from build123d import *

# Parameters (mm, degrees)
SKETCH1_R           = 16.5
SKETCH1_R_2         = 15
BOSS_EXTRUDE1_DEPTH = 40
SKETCH3_W           = 4
SKETCH3_H           = 8
CUT_EXTRUDE1_DEPTH  = 47.308746474


with BuildPart() as part:
    # Sketch1 → Boss-Extrude1 (new, symmetric)
    with BuildSketch(Plane.XY):
        Circle(SKETCH1_R)
        Circle(SKETCH1_R_2, mode=Mode.SUBTRACT)
    extrude(amount=BOSS_EXTRUDE1_DEPTH, both=True)

    # Sketch3 → Cut-Extrude1 (cut, through all)
    with BuildSketch(Plane(origin=(0, 0, 0), x_dir=(0, 0, -1), z_dir=(1, 0, 0))):
        with Locations((-38, 0)):
            Rectangle(SKETCH3_W, SKETCH3_H)
    cut_extrude1 = extrude(amount=CUT_EXTRUDE1_DEPTH, mode=Mode.SUBTRACT)

    # Mirror1: Cut-Extrude1 across plane
    add(cut_extrude1.mirror(Plane.XY), mode=Mode.SUBTRACT)


solid = part.part
Here's how the part is built. I have some questions about the finished solid (model axes, mm). A direction names the side the tool comes from. Give positions to 0.01 mm unless a question says otherwise; leave off trailing zeros. Write each loop counter-clockwise with the first axis right and the second up, starting at its lowest first coordinate (ties: lowest second). Pieces come first, ordered by that corner, then holes. Notation, with made-up numbers: (-7, 18) -> (35, 18) arc R3 cw to (35, 22) -> close; hole circle Ø3 at (76, 57.25). An arc over 180 degrees is marked (long way). Use one line per item in the form item = value. Start each with the question number.
1. Imagine slicing it at B-B on y = 0. List the corners of the cut face in (x, z) for me, plus the area to 3 significant figures.
2. Imagine slicing it at C-C on z = -34. List the corners of the cut face in (x, y) for me, plus the area to 3 significant figures.
3. Imagine slicing it at A-A on x = 0. List the corners of the cut face in (y, z) for me, plus the area to 3 significant figures.
4. Thinking about a two-plate mould opening in X: for faces 1 (the face through (-14.985, 0.66, -0.56)), 2 (the face through (-15, -4, -40)), 3 (the face through (15.24, -6.32, 0.56)), which applies, +X half, -X half, draft (parallel to the pull), parting line (faces both ways), or undercut?
5. If I drill on L1, parallel to Y at x = 0, z = 2; L2, parallel to Y at x = -9, z = -4; L3, parallel to X at y = -2.5, z = 21.5, over which ranges is the centre line in solid material (lowest first)?
6. On a 3-axis mill with a long thin cutter (end or side, diameter ignored), from which of +Z, -Z, +X, -X, +Y, -Y can I reach the whole of each face in a straight line? I mean faces 4 (the face through (-15, -4, 40)), 5 (the face through (15, 4, 38)), 6 (the face through (15.5, -0.1, -36)). Say none if no direction works.
7. Will these pins go through, and if not, where does the flat tip stop? pin 1 Ø0.5 at (x, z) = (15.5, 37.5) entering from +Y; pin 2 Ø8 at (y, z) = (-8.5, 27.5) entering from +X; pin 3 Ø1.2 at (x, z) = (15.5, -37.5) entering from +Y.
Entries:
q1.outline = (-16.5, -40) -> (-15, -40) -> (-15, 40) -> (-16.5, 40) -> close; (15, -36) -> (16.5, -36) -> (16.5, 36) -> (15, 36) -> close
q1.area = 228 mm²
q2.outline = circle Ø33 at (0, 0); hole circle Ø30 at (0, 0)
q2.area = 148 mm²
q3.outline = (-16.5, -40) -> (-15, -40) -> (-15, 40) -> (-16.5, 40) -> close; (15, -40) -> (16.5, -40) -> (16.5, 40) -> (15, 40) -> close
q3.area = 240 mm²
q4.face_1 = undercut
q4.face_2 = draft
q4.face_3 = parting line
q5.L1 = -16.5 to -15, 15 to 16.5
q5.L2 = -13.83 to -12, 12 to 13.83
q5.L3 = -16.31 to -14.79, 14.79 to 16.31
q6.face_4 = +Z, +X, -X, +Y, -Y
q6.face_5 = +Z, +X
q6.face_6 = -Z, +X
q7.pin_1 = 6.3
q7.pin_2 = 15.87
q7.pin_3 = 7.09
